Geometry: see drawing. Coordinates: mm, zero at the bounding-box minimum. A direction names the side the tool comes from. Round coordinates to 2 decimals unless told otherwise and drop trailing zeros. Order: outer loops, then holes, each group sorted by start corner. A loop starts at its lowest first (then second) coordinate and runs counter-clockwise, first axis right, second up. Notation, with made-up numbers: M 86.5,32.25 L 102.5,32.25 A24 cw 102.5,65.25 Z; hole C 14.25,-9.75 d8. An arc over 180 degrees is marked long. Answer in a Markdown table with one row per item. Add a question column.
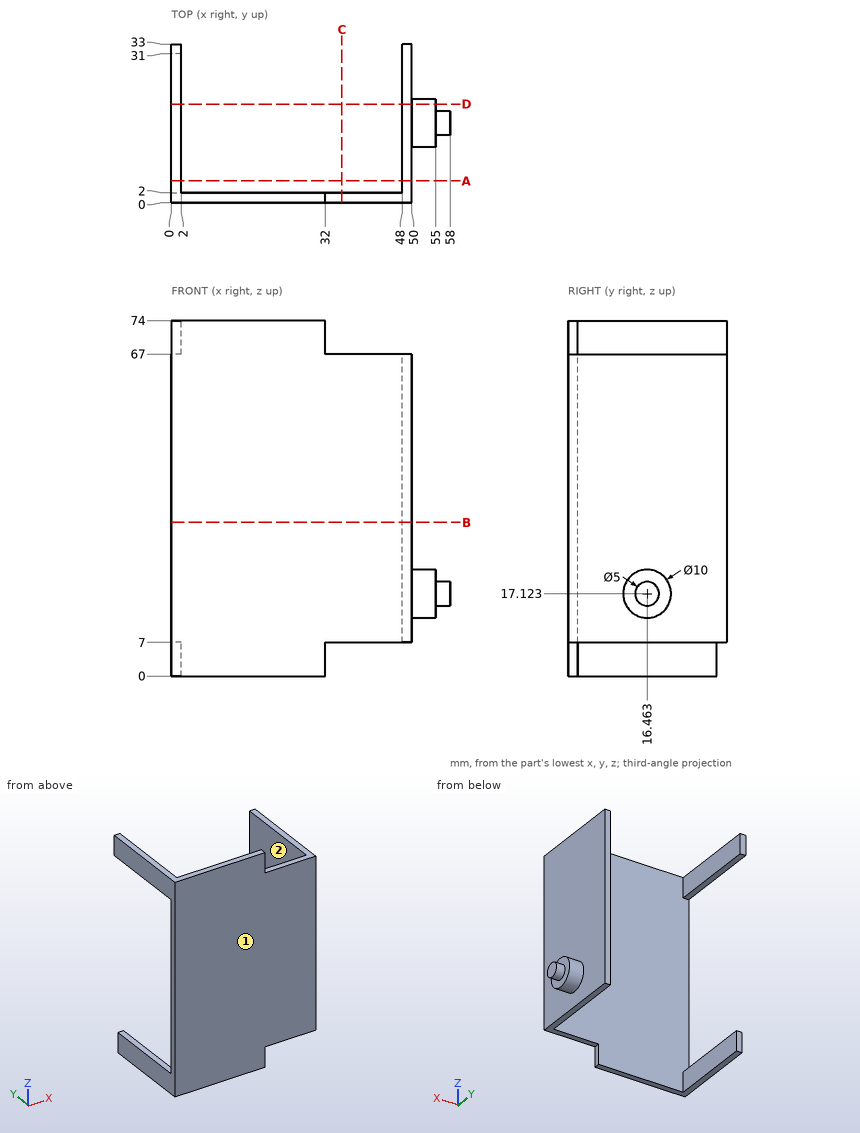
(1) Cut plane A-A (y = 4.5). Return loops of the section in (x, z).
(2) Cut plane C-C (x = 35.5). Return loops of the section in (y, z), and give its area (3 significant figures).
(3) Access query for the marked faces 1 and 2. Directions: +Z, -Z, +X, -X, +Y, -Y. A direction counts if a zero-diameter tool reaches every point of the face in a straight line with its end or side. Return the directions, or none.
(4) Line query: line 1 (X direction, y = 17, z = 14.5); line 2 (X direction, y = 22.5, z = 51.5); line 3 (Y direction, x = 47.5, z = 54). Output: solid intervals per line, ascending. Write a range as from..to.
(5) Cut plane D-D (y = 20.5). Return loops of the section in (x, z).
(6) Cut plane B-B (z = 32). Return loops of the section in (x, y).
(7) Pin query (flat end, axial travel): pin 1 (0.6 mm diameter, centred on x = 0.5, z = 4.5, fed in from +Y); pin 2 (5.5 mm diameter, centred on y = 12.5, z = 70, fed in from +X); pin 3 (3 mm diameter, centred on x = 27, z = 52, fed in from -Y); pin 4 (3 mm diameter, centred on y = 16, z = 60.5, fed in from -X). Return the tip coordinate at first contact, or that it passes through.
Answer list:
| question | item | result |
|---|---|---|
| 1 | outline | M 0,0 L 2,0 L 2,7 L 0,7 Z; M 0,67 L 2,67 L 2,74 L 0,74 Z; M 48,7 L 50,7 L 50,67 L 48,67 Z |
| 2 | outline | M 0,7 L 2,7 L 2,67 L 0,67 Z |
| 2 | area | 120 mm² |
| 3 | face 1 | +Z, -Z, +X, -X, -Y |
| 3 | face 2 | +Z, -Z, -X, +Y |
| 4 | line 1 | 48..55 |
| 4 | line 2 | 48..50 |
| 4 | line 3 | 0..2 |
| 5 | outline | M 0,0 L 2,0 L 2,7 L 0,7 Z; M 0,67 L 2,67 L 2,74 L 0,74 Z; M 48,7 L 50,7 L 50,14.17 L 55,14.17 L 55,20.07 L 50,20.07 L 50,67 L 48,67 Z |
| 6 | outline | M 0,0 L 50,0 L 50,33 L 48,33 L 48,2 L 0,2 Z |
| 7 | pin 1 | y = 31 |
| 7 | pin 2 | x = 2 |
| 7 | pin 3 | y = 0 |
| 7 | pin 4 | x = 48 |
